Check sheet for the drawn part. Datum: minimum x, y, z corner. Units: mm. Round coordinates to 2 decimals unless told otherwise and drop trailing zeros. Write each loop counter-clockwise with the first axis right and the second up, starting at its lowest first coordinate (ties: lowest second). Pieces come first, ordered by that corner, then holes. Notation, with made-up numbers: (39, 37.25) - (57, 37.25) arc R9 cw to (57, 46.25) - close; hole circle Ø7 at (41.25, 81.25). An arc over 180 degrees is marked (long way). Return JSON: item names as keys, results as strings. Group by question number.
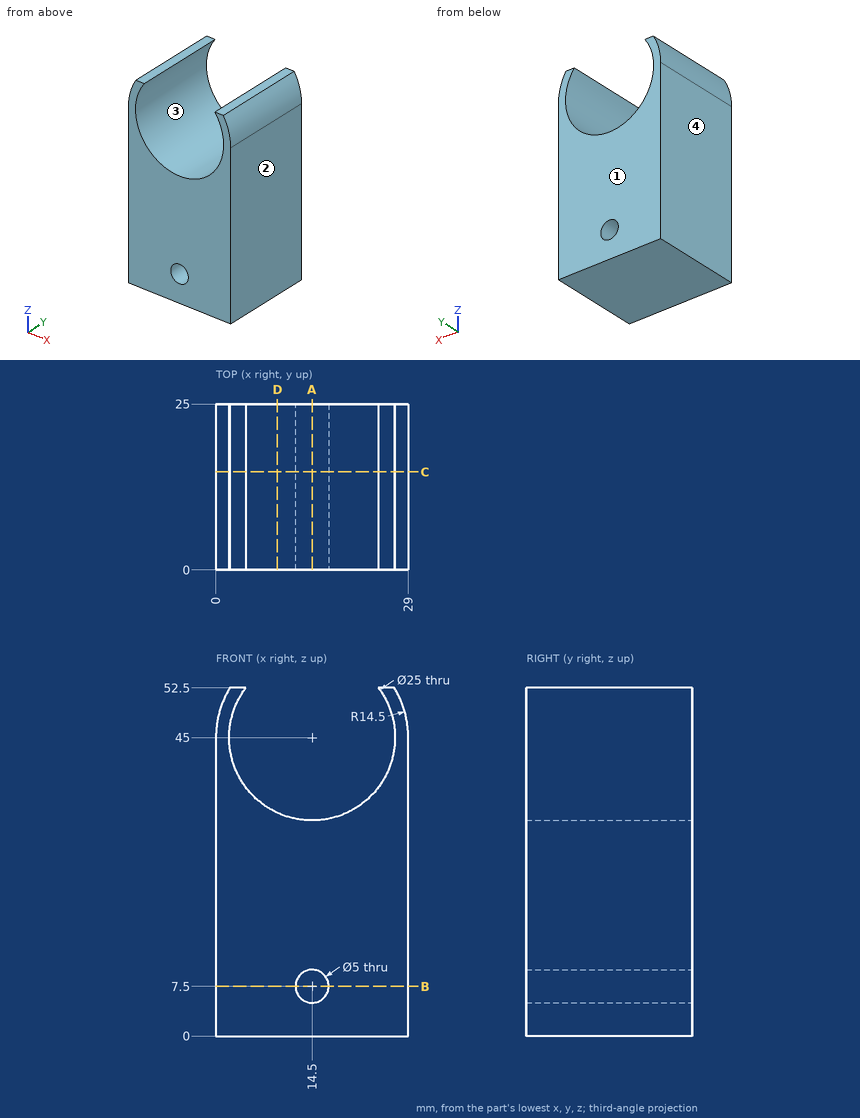
1. Section check B-B (z = 7.5). Enter the section's corners in (x, y).
2. Mould release check, pull along X, two halves, no side actions. Record for the marked faces 1, 2, 3 and 4: pulls with the +X half, pulls with the -X half, needs draft (parallel to the pull), parting line crosses it, or undercut.
3. Section check A-A (x = 14.5). Enter the section's corners in (y, z), and give its area (4 significant figures).
4. Material ranges on line 1 along Z through (x, y) = (5.5, 16.5); line 2 along X through (y, z) = (12.25, 48); line 3 along Z through (x, y) = (17.5, 15), recorded low to high.
5. Section check D-D (x = 9.25). Enter the section's corners in (y, z).
6. Section check C-C (y = 14.75). Enter the section's corners in (x, z), and give its area (3 significant figures).
Result sheet:
{
 "1": {"outline": "(0, 0) - (12, 0) - (12, 25) - (0, 25) - close; (17, 0) - (29, 0) - (29, 25) - (17, 25) - close"},
 "2": {"face 1": "needs draft", "face 2": "pulls with the +X half", "face 3": "undercut", "face 4": "pulls with the -X half"},
 "3": {"outline": "(0, 0) - (25, 0) - (25, 5) - (0, 5) - close; (0, 10) - (25, 10) - (25, 32.5) - (0, 32.5) - close", "area": "687.5 mm²"},
 "4": {"line 1": "z = 0 to 36.33", "line 2": "x = 0.31 to 2.37, 26.63 to 28.69", "line 3": "z = 0 to 32.87"},
 "5": {"outline": "(0, 0) - (25, 0) - (25, 33.66) - (0, 33.66) - close"},
 "6": {"outline": "(0, 0) - (29, 0) - (29, 45) arc R14.5 ccw to (26.91, 52.5) - (24.5, 52.5) arc R12.5 cw (long way) to (4.5, 52.5) - (2.09, 52.5) arc R14.5 ccw to (0, 45) - close; hole circle Ø5 at (14.5, 7.5)", "area": "1,070 mm²"}
}
